Input: part model. Units: mm. Frame: model coordinates. Face numbers are marked on the shaded views. Round coordinates to 2 decimals unless told otherwise and drop trailing zeros. Loops run counter-clockwise (first coordinate to the right, second up) from the corner with the lowest first, then second, coordinate; pieces in that order, holes last. Notation, with made-up numbers: (68.25, 6) -> (78.25, 6) arc R27 cw to (78.25, 40) -> close; hole circle Ø10 at (41.5, -9). An arc over 180 degrees is marked (long way). One line per question, with ' | ' between items. Start each with the question number.
Q1. Material intervals for L1, parallel to Y at x = 0, z = 2.85 (3 decimals); L2, parallel to Y at x = 15, z = 5; L3, parallel to Y at x = -13.5, z = 4.5, sorted ascending.
Q2. Cut plane A-A on y = 0. Return loops of the section in (x, z), and give its area (3 significant figures).
Q3. Cut plane B-B on z = 4.25. State how many separate pieces and enclosed holes the cut face has, and give its area (3 significant figures).
Q4. Contact query for flat-ended pins moving along their axis: P1, Ø2, axis at x = 18.5, z = 0.5, coming from the -Y side; P2, Ø1.5, axis at y = -21.5, z = 2, coming from the +X side; P3, Ø1.4, axis at y = -29, z = 3, coming from the -X side. Output: stop coordinate, or through.
Q5. Mould query, pull axis Y, two halves, no side actions, for the marked faces 1, 2, 3 and 4. Classes: pulls with the +Y half, pulls with the -Y half, needs draft (parallel to the pull), parting line crosses it, or undercut.
from build123d import *

# Parameters (mm, degrees)
SKETCH_1_R          = 31.75
EXTRUDE_1_DEPTH     = 6
SKETCH_2_W          = 10
SKETCH_2_H          = 10
CUT_EXTRUDE_1_DEPTH = 7
M2_5X0_451_D        = 2.05
M3X0_51_D           = 2.5
SKETCH_8_R          = 6.3
CUT_EXTRUDE_2_DEPTH = 7
CHAMFER_1_SIZE      = 1


with BuildPart() as part:
    # Эскиз1 → Бобышка-Вытянуть1 (new body)
    with BuildSketch(Plane.XY):
        Circle(SKETCH_1_R)
    extrude(amount=EXTRUDE_1_DEPTH)

    # Эскиз2 → Вырез-Вытянуть1 (cut, through all)
    with BuildSketch(Plane.XY.offset(6)):
        with Locations((0, -31.75)):
            Rectangle(SKETCH_2_W, SKETCH_2_H)
    extrude(amount=-CUT_EXTRUDE_1_DEPTH, mode=Mode.SUBTRACT)

    # Отверстие обработанное метчиком M2.5x0.451 (through all)
    with Locations(Plane.XY.offset(6)):
        with Locations((0, 16), (13.856406461, -8), (-13.856406461, -8)):
            Hole(M2_5X0_451_D / 2)

    # Отверстие обработанное метчиком M3x0.51 (through all)
    with Locations(Plane.XY.offset(6)):
        with Locations((-15.556349186, 15.556349186), (-15.556349186, -15.556349186), (15.556349186, -15.556349186), (15.556349186, 15.556349186), (8.838834765, 8.838834765), (-8.838834765, 8.838834765), (-8.838834765, -8.838834765), (8.838834765, -8.838834765)):
            Hole(M3X0_51_D / 2)

    # Эскиз8 → Вырез-Вытянуть2 (cut, through all)
    with BuildSketch(Plane.XY.offset(6)):
        Circle(SKETCH_8_R)
    extrude(amount=-CUT_EXTRUDE_2_DEPTH, mode=Mode.SUBTRACT)

    # Фаска1
    chamfer_1_edges = [part.edges().sort_by_distance(p)[0] for p in [
        (0, 31.75, 6),
    ]]
    chamfer(chamfer_1_edges, length=CHAMFER_1_SIZE)


solid = part.part
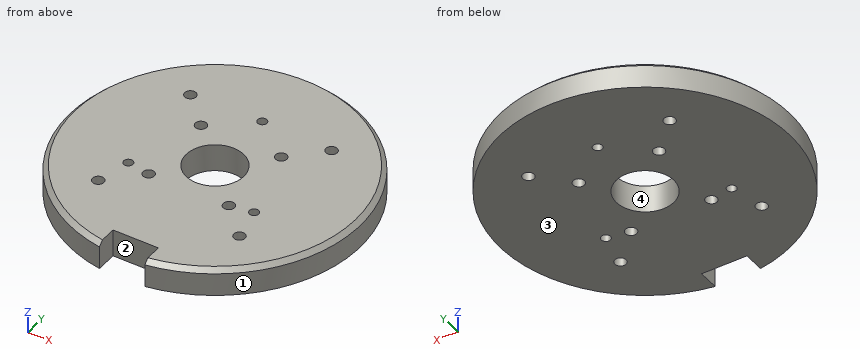
Results:
1) L1: -26.75 to -6.3, 6.3 to 14.975, 17.025 to 31.75 | L2: -27.98 to -16.68, -14.44 to 14.44, 16.68 to 27.98 | L3: -28.74 to -8.96, -7.04 to 28.74
2) outline: (-31.75, 0) -> (-6.3, 0) -> (-6.3, 6) -> (-30.75, 6) -> (-31.75, 5) -> close; (6.3, 0) -> (31.75, 0) -> (31.75, 5) -> (30.75, 6) -> (6.3, 6) -> close | area: 304 mm^2
3) separate pieces: 1 | enclosed holes: 12 | area: 2,940 mm^2
4) P1: y = -26.49 | P2: x = 24.03 | P3: x = -14.39
5) face 1: parting line crosses it | face 2: pulls with the -Y half | face 3: needs draft | face 4: undercut
